from build123d import *

# Parameters (mm, degrees)
F0_W     = 600
F0_H     = 100
F1_DEPTH = 50
F2_R     = 5
F3_DEPTH = 50.001


with BuildPart() as f1:
    # F0 (on Front) → F1 (new body)
    with BuildSketch(Plane.XZ):
        Rectangle(F0_W, F0_H)
    extrude(amount=F1_DEPTH)

    # F2 (on face) → F3 (cut, through all)
    with BuildSketch(Plane.XZ.offset(50)):
        with Locations((-275, 25)):
            Circle(F2_R)
        with Locations((-275, -25)):
            Circle(F2_R)
        with Locations((275, 25)):
            Circle(F2_R)
        with Locations((275, -25)):
            Circle(F2_R)
    extrude(amount=-F3_DEPTH, mode=Mode.SUBTRACT)


solid = f1.part
The model under review builds one solid part; all positions refer to its coordinate system, in mm. Give positions to 0.01 mm unless a question says otherwise; leave off trailing zeros. Write each loop counter-clockwise with the first axis right and the second up, starting at its lowest first coordinate (ties: lowest second). Pieces come first, ordered by that corner, then holes. Notation, with made-up numbers: M -34.75,-7 L -8.75,-7 A22 cw -8.75,4 Z; hole C 3.5,33.25 d5. An arc over 180 degrees is marked long. One line per question, with ' | ' between items. Start each with the question number.
Item 1: For pin 1 (11.5 mm diameter, centred on x = 275, z = 25, fed in from +Y), flat-tipped, find the tip position at first contact; note if it passes through.
Item 2: Wall thickness on line 1 (Z direction, x = -275, y = -24); line 2 (X direction, y = -24, z = -29.5); line 3 (X direction, y = -4.5, z = 28): over which ranges is each line inside the solid? List them lowest first. Write a range as from..to.
Item 3: Draft analysis for pull direction X (two halves, no side actions). For faces 1 (the flat face through (-300, -25, -1)), 2 (the cylindrical face through (-270.381, -25.35, -26.915)), 3 (the flat face through (-4, -25, -50)), state which applies: released by +X, released by -X, zero draft, split by the parting line, or undercut.
Item 4: We need section A-A on x = 275. Write out the cut boundary in (y, z).
Results found:
1) pin 1: stops at y = 0
2) line 1: z = -50..-30, -20..20, 30..50 | line 2: x = -300..-277.18, -272.82..272.82, 277.18..300 | line 3: x = -300..-279, -271..271, 279..300
3) face 1: released by -X | face 2: undercut | face 3: zero draft
4) outline: M -50,-50 L 0,-50 L 0,-30 L -50,-30 Z; M -50,-20 L 0,-20 L 0,20 L -50,20 Z; M -50,30 L 0,30 L 0,50 L -50,50 Z
